Verification items for the finished model (mm, model axes). Coordinates: 2 decimals unless noted, no trailing zeros. Write each loop counter-clockwise with the first axis right and the second up, starting at its lowest first coordinate (ties: lowest second). Pieces come first, ordered by that corner, then holes. Notation, with made-up numbers: (39.25, -18.75) -> (84.25, -18.75) arc R12 cw to (84.25, 3.25) -> close; hole circle Ø5 at (66.5, 63). An arc over 180 degrees is marked (long way). Use CSV: the item, a comma, the result in double quotes.
```python
from build123d import *

# Parameters (mm, degrees)
F0_W     = 100
F0_H     = 80
F0_R     = 20
F1_DEPTH = 25
F2_R     = 5


with BuildPart() as f1:
    # F0 (on Front) → F1 (new body)
    with BuildSketch(Plane.XZ):
        Rectangle(F0_W, F0_H)
        Circle(F0_R, mode=Mode.SUBTRACT)
    extrude(amount=F1_DEPTH)

    # F2
    f2_edges = [f1.edges().sort_by_distance(p)[0] for p in [
        (50, -12.5, -40),
        (50, -12.5, 40),
        (50, 0, 0),
        (50, -25, 0),
        (-50, -12.5, 40),
        (0, 0, 40),
        (0, -25, 40),
        (-50, -12.5, -40),
        (-50, 0, 0),
        (-50, -25, 0),
        (0, 0, -40),
        (0, -25, -40),
    ]]
    fillet(f2_edges, radius=F2_R)


solid = f1.part
```
1) Cross-section at B-B (z = 16). Record the boundary of the cut face in (x, y), plus the area to 3 significant figures.
Return value:
outline,"(-50, -20) arc R5 ccw to (-45, -25) -> (-12, -25) -> (-12, 0) -> (-45, 0) arc R5 ccw to (-50, -5) -> close; (12, -25) -> (45, -25) arc R5 ccw to (50, -20) -> (50, -5) arc R5 ccw to (45, 0) -> (12, 0) -> close"
area,"1,880 mm2"
2) Gauge pin test, flat end, axial feed: pin 1 (8 mm diameter, centred on x = 31, z = -28.5, fed in from +Y). Record the tip position at first contact, or that the pin passes through.
Return value:
pin 1,"y = 0"
3) Cross-section at A-A (x = 0). Record the boundary of the cut face in (y, z).
Return value:
outline,"(-25, -35) arc R5 ccw to (-20, -40) -> (-5, -40) arc R5 ccw to (0, -35) -> (0, -20) -> (-25, -20) -> close; (-25, 20) -> (0, 20) -> (0, 35) arc R5 ccw to (-5, 40) -> (-20, 40) arc R5 ccw to (-25, 35) -> close"
4) Cross-section at C-C (y = -7.25). Record the boundary of the cut face in (x, z), plus the area to 3 significant figures.
Return value:
outline,"(-50, -35) arc R5 ccw to (-45, -40) -> (45, -40) arc R5 ccw to (50, -35) -> (50, 35) arc R5 ccw to (45, 40) -> (-45, 40) arc R5 ccw to (-50, 35) -> close; hole circle Ø40 at (0, 0)"
area,"6,720 mm2"
5) Scan lines: L1, parallel to Z at x = 0, y = -18; L2, parallel to X at y = -21.75, z = 8; L3, parallel to Z at x = -17.5, y = -20. Record each from-to range of solid material in increasing order.
Return value:
L1,"-40 to -20, 20 to 40"
L2,"-49.68 to -18.33, 18.33 to 49.68"
L3,"-40 to -9.68, 9.68 to 40"
